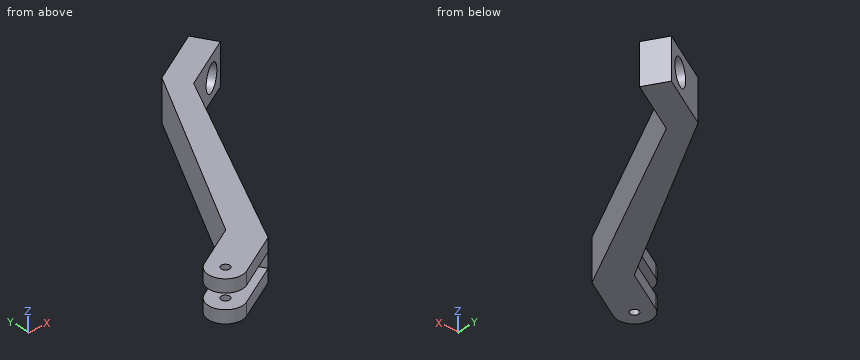
Autodesk Inventor part; units mm, degrees
ref_plane "YZ Plane" through (0, 0, 0) normal (1, 0, 0) x (0, 1, 0)
ref_plane "XZ Plane" through (0, 0, 0) normal (0, 1, 0) x (-1, 0, 0)
ref_plane "XY Plane" through (0, 0, 0) normal (0, 0, 1) x (1, 0, 0)
sketch "Sketch1" plane through (0, 0, 0) normal (0, 0, 1) x (1, 0, 0)
  circle A0 centre (0, -7.23) radius 0.5
  circle A1 centre (0, -7.23) radius 2
  point P0 (0, 0)
  dimension "d0" = 4
extrude "Extrusion1" add sketch "Sketch1" along normal blind 1.5
sketch "Sketch2" plane through (0, -7.23, 1.5) normal (0, 0, 1) x (1, 0, 0)
  circle A0 centre (0, 0) radius 2
  circle A1 centre (0, 0) radius 0.5
  circle A2 centre (0, 0) radius 2
  line L0 (1, -1.7321) -> (6.1962, 1.2679)
  line L1 (-1, 1.7321) -> (4.1962, 4.7321)
  line L2 (22.8311, 17.6353) -> (-6.9601, 0.4353) construction
  circle A3 centre (0, 0) radius 2
  line L3 (4.1962, 4.7321) -> (17.0361, 27.9727)
  line L4 (6.1962, 1.2679) -> (18.5361, 25.3746)
  line L5 (4.1962, 4.7321) -> (6.1962, 1.2679) construction
  line L6 (18.5361, 25.3746) -> (17.0361, 27.9727)
  line L7 (15.8361, 30.0512) -> (18.5361, 25.3746) construction
  point P0 (0, 7.23)
  point P1 (-1, 1.7321)
  point P2 (1, -1.7321)
  dimension "d4" = 6
  dimension "d13" = 3
extrude "Extrusion2" add sketch "Sketch2" against normal blind 1.5 contours A0 L1 L3 L6 L4 L0
ref_plane "Work Plane1" through (0, 0, -1.75) normal (0, 0, -1) x (-1, 0, 0)
sketch "Sketch3" plane through (0, 0, -1.75) normal (0, 0, -1) x (-1, 0, 0)
  line L0 (1, -5.4979) -> (-4.1962, -2.4979)
  line L1 (-4.1962, -2.4979) -> (-17.0361, 20.7427)
  line L2 (-17.0361, 20.7427) -> (-18.5361, 18.1446)
  line L3 (-18.5361, 18.1446) -> (-6.1962, -5.9621)
  line L4 (-6.1962, -5.9621) -> (-1, -8.9621)
  arc A0 (-1, -8.9621) -> (1, -5.4979) centre (0, -7.23) ccw
  circle A1 centre (0, -7.23) radius 0.5
  point P0 (0, 0)
extrude "Extrusion3" add sketch "Sketch3" along normal blind 1.5
sketch "Sketch4" plane through (0, 0, 0) normal (0, 0, -1) x (-1, 0, 0)
  line L0 (-17.0361, 20.7427) -> (-18.5361, 18.1446)
  line L1 (-18.5361, 18.1446) -> (-6.1962, -5.9621)
  line L2 (-6.1962, -5.9621) -> (-1, -8.9621)
  arc A0 (-1, -8.9621) -> (1, -5.4979) centre (0, -7.23) ccw
  line L3 (1, -5.4979) -> (-4.1962, -2.4979)
  line L4 (-4.1962, -2.4979) -> (-17.0361, 20.7427)
  circle A1 centre (0, -7.23) radius 0.5
  line L5 (1, -5.4979) -> (-4.1962, -2.4979)
  line L6 (-4.1962, -2.4979) -> (-6.1962, -5.9621)
  point P0 (0, 0)
extrude "Extrusion4" add sketch "Sketch4" along normal up to next contours L4 L6 L1 L0
sketch "Sketch5" plane through (18.5361, 18.1446, 1.5) normal (0.866, 0.5, 0) x (0, 0, -1)
  line L0 (0, 0) -> (0, 3)
  line L1 (0, 0) -> (4.75, 0)
  line L2 (4.75, 3) -> (4.75, 0)
  line L3 (0, 3) -> (4.75, 3)
  point P0 (1.5, -6.4457)
extrude "Extrusion5" add sketch "Sketch5" along normal blind 7.5
sketch "Sketch6" plane through (18.5361, 18.1446, -3.25) normal (0.5, -0.866, 0) x (0.866, 0.5, 0)
  line L0 (0, 4.75) -> (0, 0)
  line L1 (0, 0) -> (7.5, 0)
  line L2 (7.5, 4.75) -> (7.5, 0)
  line L3 (0, 4.75) -> (7.5, 4.75)
  circle A0 centre (5, 2.375) radius 1.5
  point P0 (-25.125, 3.25)
  point P1 (0, 2.375)
  point P2 (3.75, 0)
  dimension "d14" = 3
  dimension "d17" = 2.5
extrude "Extrusion6" cut sketch "Sketch6" against normal up to next contours A0
properties part number "Union_dedo_base"
Part model, mm, in its own coordinate system. Coordinates: 2 decimals unless noted, no trailing zeros. Write each loop counter-clockwise with the first axis right and the second up, starting at its lowest first coordinate (ties: lowest second). Pieces come first, ordered by that corner, then holes. Notation, with made-up numbers: M -8,-19 L 41,-19 A9 cw 41,-8 Z; hole C 43,6.25 d9. An arc over 180 degrees is marked long. Return JSON: item names as keys, results as strings.
1. Probe L1, parallel to Y at x = 0, z = 1.1; L2, parallel to Y at x = 4.5, z = -2; L3, parallel to Y at x = 8.75, z = -0.4. List the from-to ranges inside material, lowest first.
Determined:
{"L1": "-9.23 to -7.73, -6.73 to -4.92", "L2": "-6.94 to -1.95", "L3": "-0.97 to 5.74"}
2. Saw through at C-C, the plane y = -7.23. Write the cut outline in (x, z).
Determined:
{"outline": "M -2,-3.25 L -0.5,-3.25 L -0.5,-1.75 L -2,-1.75 Z; M -2,0 L -0.5,0 L -0.5,1.5 L -2,1.5 Z; M 0.5,-3.25 L 4,-3.25 L 4,-1.75 L 0.5,-1.75 Z; M 0.5,0 L 4,0 L 4,1.5 L 0.5,1.5 Z"}
3. Saw through at D-D, the plane x = 3.5. Write the cut outline in (y, z).
Determined:
{"outline": "M -7.52,-3.25 L -2.9,-3.25 L -2.9,-1.75 L -7.52,-1.75 Z; M -7.52,0 L -2.9,0 L -2.9,1.5 L -7.52,1.5 Z"}
4. Flat gauge pin, fed straight in: pin 1 Ø1 at (x, z) = (3, -2.5) entering from -Y. Where does the tip first touch, or does it go through?
Determined:
{"pin 1": "y = -8.1"}
5. Saw through at B-B, the plane x = 0. Write the cut outline in (y, z).
Determined:
{"outline": "M -9.23,-3.25 L -7.73,-3.25 L -7.73,-1.75 L -9.23,-1.75 Z; M -9.23,0 L -7.73,0 L -7.73,1.5 L -9.23,1.5 Z; M -6.73,-3.25 L -4.92,-3.25 L -4.92,-1.75 L -6.73,-1.75 Z; M -6.73,0 L -4.92,0 L -4.92,1.5 L -6.73,1.5 Z"}
